from build123d import *

# Parameters (mm, degrees)
F0_W     = 355.6
F0_H     = 228.6
F1_DEPTH = 11.938
F2_T     = -5.08
F3_R     = 2.54


with BuildPart() as f1:
    # F0 (on Top) → F1 (new body, symmetric)
    with BuildSketch(Plane.XY):
        Rectangle(F0_W, F0_H)
    extrude(amount=F1_DEPTH, both=True)

    # F2
    f2_openings = [f1.faces().sort_by_distance(p)[0] for p in [
        (0, 0, 11.938),
    ]]
    offset(amount=F2_T, openings=f2_openings)

    # F3
    f3_edges = [f1.edges().sort_by_distance(p)[0] for p in [
        (-177.8, 114.3, 0),
        (-177.8, 0, -11.938),
        (-177.8, -114.3, 0),
        (-177.8, 0, 11.938),
        (0, -114.3, -11.938),
        (177.8, -114.3, 0),
        (0, -114.3, 11.938),
        (177.8, 0, -11.938),
        (177.8, 114.3, 0),
        (177.8, 0, 11.938),
        (0, 114.3, -11.938),
        (0, 114.3, 11.938),
    ]]
    fillet(f3_edges, radius=F3_R)


solid = f1.part
Build history of the part. All positions in model axes, mm. A direction names the side the tool comes from. Round coordinates to 2 decimals unless told otherwise and drop trailing zeros. Loops run counter-clockwise (first coordinate to the right, second up) from the corner with the lowest first, then second, coordinate; pieces in that order, holes last. Notation, with made-up numbers: (-3, -23.5) -> (55, -23.5) arc R12 cw to (55, -10.5) -> close; hole circle Ø6 at (-10.75, 3.5). An arc over 180 degrees is marked (long way). One line per item, written item: value. Start each with the question number.
Q1. Probe line 1 along Y through (x, z) = (93.5, -0.25); line 2 along X through (y, z) = (22, 6.25); line 3 along Z through (x, y) = (-104.5, 16). List the from-to ranges inside material, lowest first.
Q2. Cut at A-A on z = 3.75. List the corners of the cut face in (x, y), plus the area to 3 significant figures.
Q3. Cut at B-B on y = -49. List the corners of the cut face in (x, z), plus the area to 3 significant figures.
Q4. 3-axis set-ups, long thin cutter, end or side, ignore diameter. For faces 1 (the face through (-2, 114.3, 0)), 2 (the face through (-2, 109.22, 3)): which of +Z, -Z, +X, -X, +Y, -Y reach the whole face in a straight line?
Q5. Two-plate mould, pull along X, no slides. Class faces 3 (the face through (-177.8, -2, 0)), 4 (the face through (-2, 2, -11.938)), 5 (the face through (-2, 2, -6.858)): released by +X, released by -X, zero draft, split by the parting line, or undercut.
Q6. Drop a flat-ended pin along its axis: pin 1 Ø2 at (x, y) = (-34.5, 53) entering from +Z. Give the stop position or say it passes through.
Q7. Cut at C-C on x = -92.5. List the corners of the cut face in (y, z).
Computed:
1. line 1: -114.3 to -109.22, 109.22 to 114.3
1. line 2: -177.8 to -172.72, 172.72 to 177.8
1. line 3: -11.94 to -6.86
2. outline: (-177.8, -111.76) arc R2.54 ccw to (-175.26, -114.3) -> (175.26, -114.3) arc R2.54 ccw to (177.8, -111.76) -> (177.8, 111.76) arc R2.54 ccw to (175.26, 114.3) -> (-175.26, 114.3) arc R2.54 ccw to (-177.8, 111.76) -> close; hole (-172.72, -109.22) -> (172.72, -109.22) -> (172.72, 109.22) -> (-172.72, 109.22) -> close
2. area: 5,830 mm²
3. outline: (-177.8, -9.4) arc R2.54 ccw to (-175.26, -11.94) -> (175.26, -11.94) arc R2.54 ccw to (177.8, -9.4) -> (177.8, 9.4) arc R2.54 ccw to (175.26, 11.94) -> (172.72, 11.94) -> (172.72, -6.86) -> (-172.72, -6.86) -> (-172.72, 11.94) -> (-175.26, 11.94) arc R2.54 ccw to (-177.8, 9.4) -> close
3. area: 1,990 mm²
4. face 1: +Z, -Z, +X, -X, +Y
4. face 2: +Z
5. face 3: released by -X
5. face 4: zero draft
5. face 5: undercut
6. pin 1: z = -6.86
7. outline: (-114.3, -9.4) arc R2.54 ccw to (-111.76, -11.94) -> (111.76, -11.94) arc R2.54 ccw to (114.3, -9.4) -> (114.3, 9.4) arc R2.54 ccw to (111.76, 11.94) -> (109.22, 11.94) -> (109.22, -6.86) -> (-109.22, -6.86) -> (-109.22, 11.94) -> (-111.76, 11.94) arc R2.54 ccw to (-114.3, 9.4) -> close
